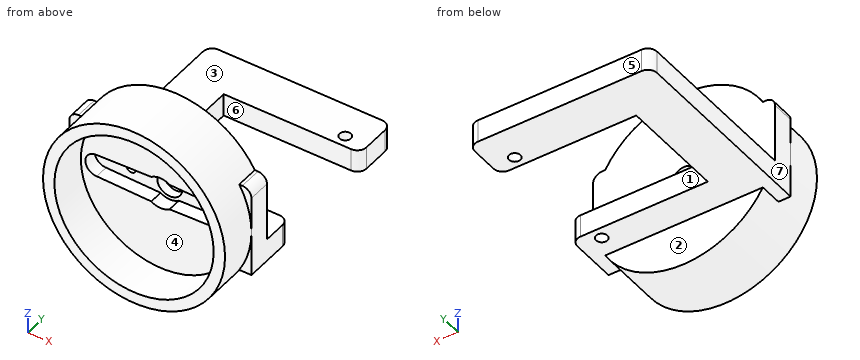
Autodesk Inventor part; units mm, degrees
ref_plane "YZ Plane" through (0, 0, 0) normal (1, 0, 0) x (0, 1, 0)
ref_plane "XZ Plane" through (0, 0, 0) normal (0, 1, 0) x (-1, 0, 0)
ref_plane "XY Plane" through (0, 0, 0) normal (0, 0, 1) x (1, 0, 0)
sketch "Sketch1" plane through (0, 0, 0) normal (0, 1, 0) x (-1, 0, 0)
  line L0 (-20, 20) -> (20, 20)
  line L1 (20, 20) -> (20, -20)
  line L2 (20, -20) -> (-20, -20)
  line L3 (-20, -20) -> (-20, 20)
  line L4 (-20, 20) -> (20, -20) construction
  line L5 (20, 20) -> (-20, -20) construction
  point P0 (0, 0)
  dimension "d0" = 40
  dimension "d1" = 40
extrude "Extrusion1" add sketch "Sketch1" along normal blind 5
sketch "Sketch4" plane through (0, 5, 0) normal (0, 1, 0) x (1, 0, 0)
  line L0 (-20, 10) -> (-10, 10)
  line L1 (-10, 10) -> (-10, 5)
  line L2 (-10, 5) -> (-20, 5)
  line L3 (-20, 5) -> (-20, 10)
  line L4 (-20, 10) -> (-10, 5) construction
  line L5 (-10, 10) -> (-20, 5) construction
  line L6 (-20, -20) -> (20, -20)
  line L7 (20, -20) -> (20, 20)
  line L8 (-20, 20) -> (-20, -20)
  point P0 (-15, 7.5)
  dimension "d20" = 10
  dimension "d21" = 5
  dimension "d23" = 25
extrude "Extrusion4" add sketch "Sketch4" along normal blind 40
sketch "Sketch8" plane through (-10, 5, -5) normal (1, 0, 0) x (0, 0, -1)
  line L0 (0, 40) -> (5, 40)
  line L1 (5, 40) -> (5, 30)
  line L2 (5, 30) -> (0, 30)
  line L3 (0, 30) -> (0, 40)
  line L4 (0, 7) -> (5, 7)
  line L5 (5, 7) -> (5, 0)
  line L6 (5, 0) -> (0, 0)
  line L7 (0, 0) -> (0, 7)
  line L8 (5, 0) -> (5, 40)
  line L9 (0, 40) -> (5, 40)
  point P0 (-5, -5)
  dimension "d44" = 5
  dimension "d45" = 10
  dimension "d46" = 5
  dimension "d47" = 7
  dimension "d48" = 23
extrude "Extrusion7" add sketch "Sketch8" along normal blind 30
sketch "Sketch9" plane through (-20, 5, -5) normal (0, 0, 1) x (1, 0, 0)
  circle A0 centre (35, 32.5) radius 1.25
  circle A1 centre (35, 4.5) radius 1.25
  line L0 (10, 30) -> (40, 30)
  line L1 (40, 40) -> (40, 30)
  line L2 (40, 7) -> (40, 0)
  point P0 (20, -5)
  dimension "d51" = 2.5
  dimension "d52" = 2.5
  dimension "d53" = 28
  dimension "d54" = 2.5
  dimension "d55" = 5
  dimension "d56" = 5
extrude "Extrusion8" cut sketch "Sketch9" against normal blind 5
sketch "Sketch11" plane through (0, 5, 0) normal (0, 1, 0) x (1, 0, 0)
  line L0 (20, -20) -> (-20, -20)
  line L1 (-20, -20) -> (-20, -10)
  line L2 (-20, -10) -> (20, -10)
  line L3 (20, -10) -> (20, -20)
  line L4 (-20, 10) -> (20, 10)
  line L5 (20, 10) -> (20, 20)
  line L6 (20, 20) -> (-20, 20)
  line L7 (-20, 20) -> (-20, 10)
  line L8 (20, 20) -> (-20, 20)
  line L9 (-20, -20) -> (20, -20)
  line L10 (20, -20) -> (20, 5)
  line L11 (20, 10) -> (20, 20)
  point P0 (0, 0)
  dimension "d59" = 40
  dimension "d60" = 10
  dimension "d61" = 40
  dimension "d62" = 10
extrude "Extrusion9" cut sketch "Sketch11" against normal blind 5
sketch "Sketch12" plane through (0, 0, 0) normal (0, -1, 0) x (1, 0, 0)
  circle A0 centre (0, 0) radius 3.5
  circle A1 centre (14, 0) radius 2.5
  circle A2 centre (-14, 0) radius 2.5
  line L0 (-20, -10) -> (20, -10)
  line L1 (-14, 2.5) -> (-2.0057, 2.8683)
  line L2 (-14, -2.5) -> (-2.0057, -2.8683)
  line L3 (14, 2.5) -> (2.0057, 2.8683)
  line L4 (14, -2.5) -> (2.0057, -2.8683)
  dimension "d65" = 7
  dimension "d66" = 5
  dimension "d67" = 5
  dimension "d68" = 14
  dimension "d69" = 10
  dimension "d70" = 10
  dimension "d71" = 14
  dimension "d72" = 12
  dimension "d73" = 12
extrude "Extrusion10" cut sketch "Sketch12" against normal blind 3
sketch "Sketch13" plane through (0, 3, 0) normal (0, -1, 0) x (1, 0, 0)
  circle A0 centre (0, 0) radius 2.75
  dimension "d76" = 5.5
extrude "Extrusion11" cut sketch "Sketch13" against normal blind 3
fillet "Fillet1" radius 2 6 edges at (20, 45, -7.5) (20, 35, -7.5) (20, 12, -7.5) (20, 2.5, 10) (-20, 2.5, 10) (-20, 45, -7.5)
sketch "Sketch14" plane through (0, 0, 0) normal (0, -1, 0) x (1, 0, 0)
  circle A0 centre (0, 0) radius 17.5
  circle A1 centre (0, 0) radius 20
  dimension "d80" = 35
  dimension "d81" = 40
extrude "Extrusion12" add sketch "Sketch14" along normal blind 8.5
sketch "Sketch15" plane through (0, 0, 0) normal (0, -1, 0) x (1, 0, 0)
  circle A0 centre (0, 0) radius 17.5
  arc A1 (2.0057, 2.8683) -> (-2.0057, 2.8683) centre (0, 0) ccw
  line L0 (2.0057, 2.8683) -> (14, 2.5)
  arc A2 (14, -2.5) -> (14, 2.5) centre (14, 0) ccw
  line L1 (14, -2.5) -> (2.0057, -2.8683)
  arc A3 (-2.0057, -2.8683) -> (2.0057, -2.8683) centre (0, 0) ccw
  line L2 (-2.0057, -2.8683) -> (-14, -2.5)
  arc A4 (-14, 2.5) -> (-14, -2.5) centre (-14, 0) ccw
  line L3 (-14, 2.5) -> (-2.0057, 2.8683)
  arc A5 (14.3614, -10) -> (14.3614, 10) centre (0, 0) ccw
  line L4 (14.3614, 10) -> (-14.3614, 10)
  arc A6 (-14.3614, 10) -> (-14.3614, -10) centre (0, 0) ccw
  line L5 (-14.3614, -10) -> (14.3614, -10)
  circle A7 centre (0, 0) radius 20
  point P0 (14.3614, 10)
extrude "Extrusion13" add sketch "Sketch15" against normal blind 5 contours L4 A0 | A0 L5 | A7
sketch "Sketch16" plane through (0, 5, 0) normal (0, 1, 0) x (1, 0, 0)
  circle A0 centre (8.45, 0) radius 1.05
  circle A1 centre (-8.45, 0) radius 1.05
  point P0 (0, 0)
  dimension "d86" = 2.1
  dimension "d87" = 2.1
extrude "Extrusion14" cut sketch "Sketch16" against normal through all
properties part number "head_bottom"
Design review of the part built by this model. Coordinates are the model's own, in mm. Face numbers are marked on the shaded views. A direction names the side the tool comes from. Coordinates: 2 decimals unless noted, no trailing zeros. Order: outer loops, then holes, each group sorted by start corner. A loop starts at its lowest first (then second) coordinate and runs counter-clockwise, first axis right, second up. Notation, with made-up numbers: M 38.25,85.25 L 68.25,85.25 A33 ccw 68.25,119.25 Z; hole C 47,-23 d3. An arc over 180 degrees is marked long. Use a Markdown table: item, result.
(1) Draft analysis for pull direction Y (two halves, no side actions). For the marked faces 5, 6 and 7, state which applies: released by +Y, released by -Y, zero draft, split by the parting line, or undercut.
Worked answers:
| item | result |
|---|---|
| face 5 | released by +Y |
| face 6 | undercut |
| face 7 | zero draft |
(2) Add section C-C (y = -4.5). Give the boundary of the cut face in (x, z).
Worked answers:
| item | result |
|---|---|
| outline | C 0,0 d40; hole C 0,0 d35 |
(3) Add section B-B (x = 10.5). Give the boundary of the cut face in (y, z).
Worked answers:
| item | result |
|---|---|
| outline | M -8.5,-17.02 L 5,-17.02 L 5,-10 L 12,-10 L 12,-5 L 5,-5 L 5,17.02 L -8.5,17.02 L -8.5,14 L 0,14 L 0,2.61 L 3,2.61 L 3,-2.61 L 0,-2.61 L 0,-14 L -8.5,-14 Z; M 35,-10 L 45,-10 L 45,-5 L 35,-5 Z |
(4) Add section D-D (z = 14.5). Give the boundary of the cut face in (x, y).
Worked answers:
| item | result |
|---|---|
| outline | M -13.77,-8.5 L -9.8,-8.5 L -9.8,0 L 9.8,0 L 9.8,-8.5 L 13.77,-8.5 L 13.77,5 L -13.77,5 Z |
(5) Add section A-A (x = 0). Give the boundary of the cut face in (y, z), then the cut area to 4 significant figures.
Worked answers:
| item | result |
|---|---|
| outline | M -8.5,-20 L 5,-20 L 5,-10 L 12,-10 L 12,-5 L 5,-5 L 5,-2.75 L 3,-2.75 L 3,-3.5 L 0,-3.5 L 0,-17.5 L -8.5,-17.5 Z; M -8.5,17.5 L 0,17.5 L 0,3.5 L 3,3.5 L 3,2.75 L 5,2.75 L 5,20 L -8.5,20 Z; M 35,-10 L 45,-10 L 45,-5 L 35,-5 Z |
| area | 295.5 mm2 |
(6) For P1, Ø1.3, axis at x = -8.45, z = 0, coming from the -Y side; P2, Ø5.5, axis at x = 3, z = 0.5, coming from the -Y side; P3, Ø2.5, axis at x = 8.45, z = 0, coming from the -Y side; P4, Ø1.5, axis at x = -0.5, y = 7.5, coming from the -Z side, all flat-tipped, find the tip position at first contact; note any pin that passes through.
Worked answers:
| item | result |
|---|---|
| P1 | passes through |
| P2 | stops at y = 0 |
| P3 | stops at y = 3 |
| P4 | stops at z = -10 |
(7) Wall thickness on probe 1 along Z at (x, y) = (0, -5); probe 2 along Y at (x, z) = (-2, -9.5): over which ranges is each line inside the solid? List them lowest first.
Worked answers:
| item | result |
|---|---|
| probe 1 | z = -20 to -17.5, 17.5 to 20 |
| probe 2 | y = 0 to 12, 35 to 45 |
(8) For the marked faces 1, 2, 3 and 4, list the 3-axis set-ups (+Z, -Z, +X, -X, +Y, -Y) from which the entire face can be reached by the end or side of a thin tool; tool diameter is ignored.
Worked answers:
| item | result |
|---|---|
| face 1 | +Z, -Z, +X |
| face 2 | -Z, +X, -X, +Y |
| face 3 | +Z, +X, -X, +Y |
| face 4 | -Y |
